from build123d import *

# Parameters (mm, degrees)
REVOLVE_1_ANGLE          = 40
SKETCH_4_W               = 4.8
SKETCH_4_H               = 4.8
EXTRUDE_1_DEPTH          = 6
SKETCH_7_R               = 1.5
CUT_EXTRUDE_4_DEPTH      = 95.895882206
SKETCH_13_R              = 1.5
CUT_EXTRUDE_7_DEPTH      = 57.80711304
CUT_EXTRUDE_8_DEPTH      = 5
PATTERN_CIRCULAR_1_COUNT = 4
PATTERN_CIRCULAR_1_ANGLE = 15
SKETCH_10_W              = 2.2
SKETCH_10_H              = 5.2
CUT_EXTRUDE_5_DEPTH      = 3
SKETCH_11_W              = 47.375376564
SKETCH_11_H              = 32.407082742
CUT_EXTRUDE_6_DEPTH      = 149.607349927
SKETCH_12_W              = 14
SKETCH_12_H              = 30
EXTRUDE_2_DEPTH          = 5
FILLET_1_R               = 5


# Read off the part's stored shape, not the designer's step: 旋转1
with BuildPart() as part:
    # 旋转1 outline → 旋转1 (revolve)
    with BuildSketch(Plane(origin=(0, 0, 0), x_dir=(0.3420201433256701, 0, -0.9396926207859079), z_dir=(0.9396926207859079, 0, 0.3420201433256701))):
        Polygon((134, 5), (125, 5), (125, -5), (134, -5), (134, -7.5), (136.5, -10), (139, -7.5), (139, 7.5), (136.5, 10), (134, 7.5), align=None)
    revolve(axis=Axis((0, 0, 0), (0, 1, 0)), revolution_arc=REVOLVE_1_ANGLE)

    # 草图4 → 凸台-拉伸1 (add)
    with BuildSketch(Plane(origin=(0, 0, 0), x_dir=(0.3420201433256631, 0, 0.9396926207859104), z_dir=(-0.9396926207859104, 0, 0.3420201433256631))):
        with Locations((-132, 0)):
            Rectangle(SKETCH_4_W, SKETCH_4_H)
    extrude(amount=EXTRUDE_1_DEPTH)

    # 草图7 → 切除-拉伸4 (cut, through all)
    with BuildSketch(Plane(origin=(-45.967507263, 0, -126.294688234), x_dir=(-0.9396926207859105, 0, 0.3420201433256632), z_dir=(-0.3420201433256632, 0, -0.9396926207859105))):
        with Locations((3, 0)):
            Circle(SKETCH_7_R)
    extrude(amount=-CUT_EXTRUDE_4_DEPTH, mode=Mode.SUBTRACT)

    # 草图13 → 切除-拉伸7 (cut, through all)
    with BuildSketch(Plane(origin=(0, 0, -139), x_dir=(-1, 0, 0), z_dir=(0, 0, -1))):
        Circle(SKETCH_13_R)
    cut_extrude_7 = extrude(amount=-CUT_EXTRUDE_7_DEPTH, mode=Mode.SUBTRACT)

    # 草图14 → 切除-拉伸8 (cut)
    with BuildSketch(Plane(origin=(0, 0, -139), x_dir=(-1, 0, 0), z_dir=(0, 0, -1))):
        Polygon((0, -3.175426481), (2.75, -1.58771324), (2.75, 1.58771324), (0, 3.175426481), (-2.75, 1.58771324), (-2.75, -1.58771324), align=None)
    cut_extrude_8 = extrude(amount=-CUT_EXTRUDE_8_DEPTH, mode=Mode.SUBTRACT)

    # 阵列(圆周)1: 切除-拉伸7, 切除-拉伸8 ×4 about axis
    pattern_circular_1_axis = Axis((0, 0, 0), (0, 1, 0))
    add([cut_extrude_7.rotate(pattern_circular_1_axis, i * PATTERN_CIRCULAR_1_ANGLE / (PATTERN_CIRCULAR_1_COUNT - 1)) for i in range(1, PATTERN_CIRCULAR_1_COUNT)], mode=Mode.SUBTRACT)
    add([cut_extrude_8.rotate(pattern_circular_1_axis, i * PATTERN_CIRCULAR_1_ANGLE / (PATTERN_CIRCULAR_1_COUNT - 1)) for i in range(1, PATTERN_CIRCULAR_1_COUNT)], mode=Mode.SUBTRACT)

    # 草图10 → 切除-拉伸5 (cut)
    with BuildSketch(Plane(origin=(0, 0, 0), x_dir=(0.3420201433256631, 0, 0.9396926207859104), z_dir=(-0.9396926207859104, 0, 0.3420201433256631))):
        with Locations((-137.9, 0)):
            Rectangle(SKETCH_10_W, SKETCH_10_H)
        Polygon((-127.2, 5), (-125, 5), (-123.655375964, 5), (-123.655375964, 1.8), (-125, 1.8), (-127.2, 1.8), align=None)
        Polygon((-127.2, -1.8), (-125, -1.8), (-123.655375964, -1.8), (-123.655375964, -5), (-125, -5), (-127.2, -5), align=None)
    extrude(amount=-CUT_EXTRUDE_5_DEPTH, mode=Mode.SUBTRACT)

    # 草图11 → 切除-拉伸6 (cut, through all)
    with BuildSketch(Plane(origin=(0, 0, 0), x_dir=(0, -1, 0), z_dir=(0.9990482215818578, 0, 0.0436193873653361))):
        with Locations((-1.017262687, 125.577370773)):
            Rectangle(SKETCH_11_W, SKETCH_11_H)
    extrude(amount=CUT_EXTRUDE_6_DEPTH, mode=Mode.SUBTRACT)

    # 草图12 → 凸台-拉伸2 (add)
    with BuildSketch(Plane(origin=(0, 0, 0), x_dir=(0.043619387365336125, 0, -0.9990482215818578), z_dir=(0.9990482215818577, 0, 0.04361938736533612))):
        with Locations((132, 0)):
            Rectangle(SKETCH_12_W, SKETCH_12_H)
    extrude(amount=EXTRUDE_2_DEPTH)

    # 圆角1
    fillet_1_edges = [part.edges().sort_by_distance(p)[0] for p in [
        (7.950043975, 15, -124.771979229),
        (7.950043975, -15, -124.771979229),
        (8.560715398, -15, -138.758654331),
        (8.560715398, 15, -138.758654331),
    ]]
    fillet(fillet_1_edges, radius=FILLET_1_R)


solid = part.part
Can you work these out from the model? Positions are in its coordinate system, mm. A direction names the side the tool comes from. Round coordinates to 2 decimals unless told otherwise and drop trailing zeros. Order: outer loops, then holes, each group sorted by start corner. A loop starts at its lowest first (then second) coordinate and runs counter-clockwise, first axis right, second up. Notation, with made-up numbers: (61, -23) - (90, -23) arc R21 ccw to (90, 1) - close; hole circle Ø4 at (-4, 5). An arc over 180 degrees is marked (long way). Answer in a Markdown table with one row per item.
(1) Suppose I cut it at B-B, the plane y = -11.5. Please give me the cut outline in (x, z), plus the area to 3 significant figures.
From the geometry:
| item | result |
|---|---|
| outline | (5.46, -125.11) - (6.05, -138.64) - (11.05, -138.42) - (10.46, -124.89) - close |
| area | 67.7 mm2 |
(2) If we mould it in two halves opening along Z, with no side actions, what happens to faces 6 (the face through (-2.75, 0, -137)), 7 (the face through (-42.115, -3.422, -120.035)), 8 (the face through (-45.399, -0.036, -129.056))? For each: released by +Z, released by -Z, zero draft, split by the parting line, or undercut.
From the geometry:
| item | result |
|---|---|
| face 6 | zero draft |
| face 7 | released by +Z |
| face 8 | undercut |
(3) Suppose I cut it at A-A, the plane y = 0. Count the separate pieces of the cut face and the enclosed holes in it, plus the area to 3 significant figures.
From the geometry:
| item | result |
|---|---|
| separate pieces | 6 |
| enclosed holes | 0 |
| area | 586 mm2 |
(4) Please list where these lines run through material, in increasing order: L1, parallel to X at y = 0, z = -131; L2, parallel to Y at x = 0, z = -129.5; L3, parallel to X at y = 0, z = -129.75. Write a range as from..to.
From the geometry:
| item | result |
|---|---|
| L1 | x = -44.49..-37.95, -32.25..-24.62, -21.58..-12.97, -9.96..-1.5, 1.5..10.72 |
| L2 | y = -5..-1.5, 1.5..5 |
| L3 | x = -44.03..-37.61, -33.21..-24.4, -21.36..-12.86, -9.85..-1.5, 1.5..10.67 |
(5) Which directions (+Z, -Z, +X, -X, +Y, -Y) give clear straight access to the entire face, cutting with the end or side of a thin tool? Please do faces 1 (the face through (-48, -2.4, -123)), 2 (the face through (8, 15, -132)), 3 (the face through (5.686, -9.93, -130.222)), 4 (the face through (-33.99, -2.37, -132.24)), 5 (the face through (7.915, -0.14, -124.774)).
From the geometry:
| item | result |
|---|---|
| face 1 | +Z, -X, -Y |
| face 2 | +Z, -Z, +X, -X, +Y |
| face 3 | -Y |
| face 4 | none |
| face 5 | +Z, +Y, -Y |
(6) For P1, Ø4, axis at y = -6, z = -129.5, coming from the -X side; P2, Ø0.9, axis at x = -46, z = -130, coming from the -Y side; P3, Ø4.5, axis at x = -26, z = -127, coming from the +Y side, each with a flat end and sliding along its axis, tell me the tip position at first contact or that it passes through.
From the geometry:
| item | result |
|---|---|
| P1 | stops at x = -47.54 |
| P2 | stops at y = -9.05 |
| P3 | stops at y = 5 |
